Autodesk Inventor part; units mm, degrees
ref_plane "YZ Plane" through (0, 0, 0) normal (1, 0, 0) x (0, 1, 0)
ref_plane "XZ Plane" through (0, 0, 0) normal (0, 1, 0) x (-1, 0, 0)
ref_plane "XY Plane" through (0, 0, 0) normal (0, 0, 1) x (1, 0, 0)
sketch "Sketch1" plane through (0, 0, 0) normal (1, 0, 0) x (0, 1, 0)
  line L0 (12.7, 12.2788) -> (-12.7, 12.2788)
  line L1 (-12.7, 12.2788) -> (-12.7, -13.1212)
  line L2 (-12.7, -13.1212) -> (12.7, -13.1212)
  line L3 (12.7, -13.1212) -> (12.7, 12.2788)
  line L4 (0, 32.4321) -> (0, -31.5519)
  line L5 (24.3369, 0) -> (-19.9975, 0)
  point P0 (0, 0)
  dimension "d0" = 25.4
extrude "Extrusion1" add sketch "Sketch1" along normal blind 406.4
sketch "Sketch3" plane through (406.4, 0, 0) normal (1, 0, 0) x (0, 0, -1)
  line L0 (-10.6786, 11.1125) -> (11.521, 11.1125)
  line L1 (11.521, 11.1125) -> (11.521, -11.0998)
  line L2 (11.521, -11.0998) -> (-10.6786, -11.0998)
  line L3 (-10.6786, -11.0998) -> (-10.6786, 11.1125)
  line L4 (13.1212, 12.7) -> (-12.2788, 12.7)
  line L5 (-12.2788, 12.7) -> (-12.2788, -12.7)
  line L6 (13.1212, -12.7) -> (13.1212, 12.7)
  line L7 (-12.2788, -12.7) -> (13.1212, -12.7)
  point P0 (0, 0)
  dimension "d5" = 1.5875
  dimension "d6" = 1.6002
  dimension "d7" = 1.6002
  dimension "d8" = 1.6002
extrude "Extrusion2" cut sketch "Sketch3" against normal through all contours L0 L1 L2 L3
sketch "Sketch4" plane through (0, -12.7, 12.2788) normal (0, 0, 1) x (1, 0, 0)
  circle A0 centre (381, 12.7) radius 3.175
  line L0 (406.4, 25.4) -> (406.4, 0)
  point P0 (0, 12.7)
  point P1 (406.4, 12.7)
  point P2 (406.4, 12.7)
  dimension "d11" = 6.35
  dimension "d12" = 25.4
extrude "Extrusion3" cut sketch "Sketch4" against normal through all
properties part number "Channel" material "Aluminum 6061"
Source: CAD feature listing. Evaluate the final solid. Frame: model axes, mm. A direction names the side the tool comes from. Round coordinates to 2 decimals unless told otherwise and drop trailing zeros. Loops run counter-clockwise (first coordinate to the right, second up) from the corner with the lowest first, then second, coordinate; pieces in that order, holes last. Notation, with made-up numbers: (35, -26) -> (83, -26) arc R20 cw to (83, -16) -> close; hole circle Ø9 at (76, 31.25). An arc over 180 degrees is marked (long way). Answer as a JSON object with one key per item and string values. Group by question number.
Q1. Mould query, pull axis Y, two halves, no side actions, for faces 1 (the flat face through (206, 0, 10.679)), 2 (the flat face through (200, 12.7, -1)), 3 (the flat face through (200, 0, 12.279)), 4 (the flat face through (206, 0, -11.521)). Classes: pulls with the +Y half, pulls with the -Y half, needs draft (parallel to the pull), parting line crosses it, or undercut.
Q2. Section query B-B (x = 215). Output: boundary loops of the cut face in (y, z), plus the area to 3 significant figures.
Q3. Access query for faces 5 (the flat face through (200, -12.7, 0)), 6 (the flat face through (206, 11.112, 0)). Directions: +Z, -Z, +X, -X, +Y, -Y. A direction counts if a zero-diameter tool reaches every point of the face in a straight line with its end or side. Return the directions, or none.
Q4. Contact query for a flat-ended pin moving along its axis: P1, Ø10, axis at y = -5, z = 8, coming from the +X side. Output: stop coordinate, or through.
Q5. Ray query, line 1 (Y direction, x = 381, z = -12.1) (3 decimals); line 2 (Z direction, x = 159.5, y = 7.75); line 3 (Y direction, x = 293.5, z = 8.25). Return the intervals inside material, ascending. Write a range as from..to.
Q6. Section query A-A (z = 3). Output: boundary loops of the cut face in (x, y), plus the area to 3 significant figures.
Completed:
{
 "1": {"face 1": "undercut", "face 2": "pulls with the +Y half", "face 3": "needs draft", "face 4": "undercut"},
 "2": {"outline": "(-12.7, -13.12) -> (12.7, -13.12) -> (12.7, 12.28) -> (-12.7, 12.28) -> close; hole (-11.1, -11.52) -> (11.11, -11.52) -> (11.11, 10.68) -> (-11.1, 10.68) -> close", "area": "152 mm²"},
 "3": {"face 5": "+Z, -Z, +X, -X, -Y", "face 6": "+X, -X"},
 "4": {"P1": "x = 406.4"},
 "5": {"line 1": "-12.7..-3.175, 3.175..12.7", "line 2": "-13.12..-11.52, 10.68..12.28", "line 3": "-12.7..-11.1, 11.11..12.7"},
 "6": {"outline": "(0, -12.7) -> (406.4, -12.7) -> (406.4, -11.1) -> (0, -11.1) -> close; (0, 11.11) -> (406.4, 11.11) -> (406.4, 12.7) -> (0, 12.7) -> close", "area": "1,300 mm²"}
}
